Could you check a few things on this model? Use its own coordinates, in mm. Face numbers are marked on the shaded views. A direction names the side the tool comes from. Give positions to 0.01 mm unless a question says otherwise; leave off trailing zeros. Write each loop counter-clockwise with the first axis right and the second up, starting at its lowest first coordinate (ties: lowest second). Pieces come first, ordered by that corner, then holes. Notation, with made-up numbers: (-40, 22.25) - (4, 22.25) arc R17 ccw to (4, 55.25) - close; hole circle Ø7 at (72.5, 7). An arc over 180 degrees is marked (long way). Use one line per item in the form item = value.
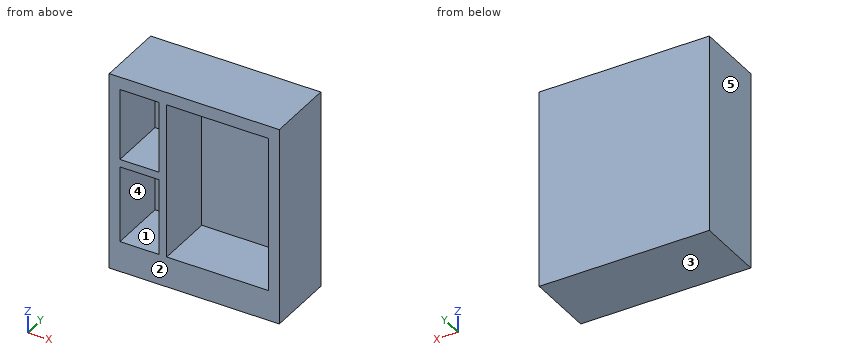
```python
from build123d import *

# Parameters (mm, degrees)
F0_W     = 1112
F0_H     = 450
F1_DEPTH = 1300
F2_W     = 972
F2_H     = 1017.5
F3_DEPTH = 380
F4_W     = 50
F4_H     = 467.5
F4_H_2   = 50
F4_W_2   = 255.950524
F4_H_3   = 500
F5_DEPTH = 380


with BuildPart() as f1:
    # F0 (on Top) → F1 (new body)
    with BuildSketch(Plane.XY):
        Rectangle(F0_W, F0_H)
    extrude(amount=-F1_DEPTH)

    # F2 (on face) → F3 (cut)
    with BuildSketch(Plane.XZ.offset(225)):
        with Locations((0, -591.25)):
            Rectangle(F2_W, F2_H)
    extrude(amount=-F3_DEPTH, mode=Mode.SUBTRACT)

    # F4 (on face) → F5 (join)
    with BuildSketch(Plane.XZ.offset(225)):
        with Locations((-205.049476, -316.25)):
            Rectangle(F4_W, F4_H)
        with Locations((-205.049476, -575)):
            Rectangle(F4_W, F4_H_2)
        with Locations((-358.024738, -575)):
            Rectangle(F4_W_2, F4_H_2)
        with Locations((-205.049476, -850)):
            Rectangle(F4_W, F4_H_3)
    extrude(amount=-F5_DEPTH)


solid = f1.part
```
1. For pin 1 (5 mm diameter, centred on x = 240.5, z = -792, fed in from -Y), with a flat end and sliding along its axis, tell me the tip position at first contact or that it passes through.
Response values:
pin_1 = 155
2. If we mould it in two halves opening along Z, with no side actions, what happens to the marked faces 3, 4 and 5? For each: pulls with the +Z half, pulls with the -Z half, needs draft (parallel to the pull), parting line crosses it, or undercut.
Response values:
face_3 = pulls with the -Z half
face_4 = undercut
face_5 = needs draft
3. If I drill on line 1 (X direction, y = -111.5, z = -422); line 2 (Z direction, x = 225.5, y = -196); line 3 (X direction, y = 35.5, z = -595), over which ranges is the centre line in solid material (lowest first)? Write a range as from..to.
Response values:
line_1 = -556..-486, -230.05..-180.05, 486..556
line_2 = -1300..-1100, -82.5..0
line_3 = -556..-180.05, 486..556
4. Which directions (+Z, -Z, +X, -X, +Y, -Y) give clear straight access to the entire face, cutting with the end or side of a thin tool? Please do the marked faces 1 and 2.
Response values:
face_1 = -Y
face_2 = +Z, -Z, +X, -X, -Y
5. Imagine slicing it at B-B, the plane y = 65.5. List the corners of the cut face in (x, z) for me.
Response values:
outline = (-556, -1300) - (556, -1300) - (556, 0) - (-556, 0) - close; hole (-486, -1100) - (-230.05, -1100) - (-230.05, -600) - (-486, -600) - close; hole (-486, -550) - (-230.05, -550) - (-230.05, -82.5) - (-486, -82.5) - close; hole (-180.05, -1100) - (486, -1100) - (486, -82.5) - (-180.05, -82.5) - close
6. Imagine slicing it at D-D, the plane x = -340. List the corners of the cut face in (y, z) for me, and give its area (3 significant figures).
Response values:
outline = (-225, -1300) - (225, -1300) - (225, 0) - (-225, 0) - (-225, -82.5) - (155, -82.5) - (155, -550) - (-225, -550) - (-225, -600) - (155, -600) - (155, -1100) - (-225, -1100) - close
area = 217,000 mm²
7. Imagine slicing it at C-C, the plane z = -983. List the corners of the cut face in (x, y) for me, and give its area (3 significant figures).
Response values:
outline = (-556, -225) - (-486, -225) - (-486, 155) - (-230.05, 155) - (-230.05, -225) - (-180.05, -225) - (-180.05, 155) - (486, 155) - (486, -225) - (556, -225) - (556, 225) - (-556, 225) - close
area = 150,000 mm²
8. Imagine slicing it at A-A, the plane x = -53.5. List the corners of the cut face in (y, z) for me, and give its area (3 significant figures).
Response values:
outline = (-225, -1300) - (225, -1300) - (225, 0) - (-225, 0) - (-225, -82.5) - (155, -82.5) - (155, -1100) - (-225, -1100) - close
area = 198,000 mm²
